from build123d import *

# Parameters (mm, degrees)
F1_DEPTH = 19.05
F3_DEPTH = 38.101
F4_R     = 2.5527
F5_DEPTH = 38.101


with BuildPart() as f1:
    # F0 (on Top) → F1 (new body, symmetric)
    with BuildSketch(Plane.XY):
        with BuildLine():
            ThreePointArc((250.825, 38.1), (233.1562165751, 80.7562165751), (190.5, 98.425))
            Line((190.5, 98.425), (-190.5, 98.425))
            ThreePointArc((-190.5, 98.425), (-233.1562165751, 80.7562165751), (-250.825, 38.1))
            Line((-250.825, 38.1), (-250.825, -38.1))
            ThreePointArc((-250.825, -38.1), (-233.1562165751, -80.7562165751), (-190.5, -98.425))
            Line((-190.5, -98.425), (190.5, -98.425))
            ThreePointArc((190.5, -98.425), (233.1562165751, -80.7562165751), (250.825, -38.1))
            Line((250.825, -38.1), (250.825, 38.1))
        make_face()
    extrude(amount=F1_DEPTH, both=True)

    # F2 (on face) → F3 (cut, through all)
    with BuildSketch(Plane.XY.offset(19.05)):
        with BuildLine():
            Line((190.5, 79.375), (-190.5, 79.375))
            ThreePointArc((-190.5, 79.375), (-219.6858323935, 67.2858323935), (-231.775, 38.1))
            Line((-231.775, 38.1), (-231.775, -38.1))
            ThreePointArc((-231.775, -38.1), (-219.6858323935, -67.2858323935), (-190.5, -79.375))
            Line((-190.5, -79.375), (190.5, -79.375))
            ThreePointArc((190.5, -79.375), (219.6858323935, -67.2858323935), (231.775, -38.1))
            Line((231.775, -38.1), (231.775, 38.1))
            ThreePointArc((231.775, 38.1), (219.6858323935, 67.2858323935), (190.5, 79.375))
        make_face()
    extrude(amount=-F3_DEPTH, mode=Mode.SUBTRACT)

    # F4 (on face) → F5 (cut, through all)
    with BuildSketch(Plane.XY.offset(19.05)):
        with Locations((-190.5, 88.9)):
            Circle(F4_R)
        with Locations((-38.1, 88.9)):
            Circle(F4_R)
        with Locations((-114.3, 88.9)):
            Circle(F4_R)
        with Locations((38.1, 88.9)):
            Circle(F4_R)
        with Locations((114.3, 88.9)):
            Circle(F4_R)
        with Locations((190.5, 88.9)):
            Circle(F4_R)
        with Locations((241.3000668421, 38.1)):
            Circle(F4_R)
        with Locations((241.3000668421, -38.1)):
            Circle(F4_R)
        with Locations((190.5, -88.9)):
            Circle(F4_R)
        with Locations((114.3, -88.9)):
            Circle(F4_R)
        with Locations((38.1, -88.9)):
            Circle(F4_R)
        with Locations((-38.1, -88.9)):
            Circle(F4_R)
        with Locations((-114.3, -88.9)):
            Circle(F4_R)
        with Locations((-190.5, -88.9)):
            Circle(F4_R)
        with Locations((-241.3, -38.1)):
            Circle(F4_R)
        with Locations((-241.3, 38.1)):
            Circle(F4_R)
    extrude(amount=-F5_DEPTH, mode=Mode.SUBTRACT)


with BuildPart() as f6_1:
    # F6: copy of F1
    add(f1.part)


solid = f1.part
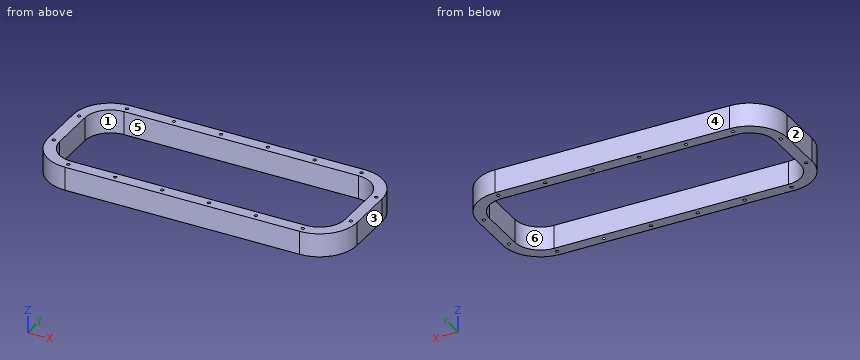
Read the model definition and answer for the solid it produces. Units are mm, in the model's axes. Face numbers are marked on the shaded views. A direction names the side the tool comes from. Coordinates: 2 decimals unless noted, no trailing zeros. Loops run counter-clockwise (first coordinate to the right, second up) from the corner with the lowest first, then second, coordinate; pieces in that order, holes last. Notation, with made-up numbers: (-31.75, -5) - (9.25, -5) arc R17 ccw to (9.25, 22) - close; hole circle Ø6 at (-25.75, 83). An arc over 180 degrees is marked (long way). Answer in a Markdown table with one row per item.
Q1. For the marked faces 1 and 2, determine the directions among +Z, -Z, +X, -X, +Y, -Y from which every point of the face is accessible in a straight line to the end or side of a thin tool.
Here are the results:
| item | result |
|---|---|
| face 1 | +Z, -Z |
| face 2 | +Z, -Z, -X, +Y, -Y |
Q2. Find section B-B on x = -99.5. Write down the section's boundary in (y, z) (3 decimals), plus the area to 3 significant figures.
Here are the results:
| item | result |
|---|---|
| outline | (-98.425, -19.05) - (-79.375, -19.05) - (-79.375, 19.05) - (-98.425, 19.05) - close; (79.375, -19.05) - (98.425, -19.05) - (98.425, 19.05) - (79.375, 19.05) - close |
| area | 1,450 mm^2 |
Q3. Find section A-A on y = 30.5. Write down the section's boundary in (x, z) (3 decimals), plus the area to 3 significant figures.
Here are the results:
| item | result |
|---|---|
| outline | (-250.825, -19.05) - (-231.775, -19.05) - (-231.775, 19.05) - (-250.825, 19.05) - close; (231.775, -19.05) - (250.825, -19.05) - (250.825, 19.05) - (231.775, 19.05) - close |
| area | 1,450 mm^2 |
Q4. Straight lines are drawn through the part: line 1 along Y through (x, z) = (-38.1, 8) (3 decimals); line 2 along Y through (x, z) = (114, -4) (3 decimals); line 3 along X through (y, z) = (34, 5) (3 decimals). For each, find the intervals that lie inside material, in ascending order. Write a range as [from, to].
Here are the results:
| item | result |
|---|---|
| line 1 | y = [-98.425, -91.453], [-86.347, -79.375], [79.375, 86.347], [91.453, 98.425] |
| line 2 | y = [-98.425, -91.435], [-86.365, -79.375], [79.375, 86.365], [91.435, 98.425] |
| line 3 | x = [-250.825, -231.775], [231.775, 250.825] |
Q5. Find section C-C on z = -12.5. Count the separate pieces of the cut face and the enclosed holes in it, plus the area to 3 significant figures.
Here are the results:
| item | result |
|---|---|
| separate pieces | 1 |
| enclosed holes | 17 |
| area | 23,200 mm^2 |
Q6. Given P1, Ø3, axis at x = 241.3, y = -38.1, coming from the -Z side; P2, Ø1, axis at y = -75, z = -10.5, coming from the +X side; P3, Ø8, axis at y = -74.5, z = -1, coming from the +X side, each flat-ended and moving along its own axis, determine where each tip first touches the part or whether it passes through.
Here are the results:
| item | result |
|---|---|
| P1 | passes through |
| P2 | stops at x = 238.61 |
| P3 | stops at x = 241.39 |
Q7. The mould has two halves that part along X. Classify the marked faces 3, 4, 5 and 6: pulls with the +X half, pulls with the -X half, needs draft (parallel to the pull), parting line crosses it, or undercut.
Here are the results:
| item | result |
|---|---|
| face 3 | pulls with the +X half |
| face 4 | needs draft |
| face 5 | undercut |
| face 6 | undercut |
